CAD build for the part. Positions are in the model's coordinates, mm. Face numbers are marked on the shaded views. A direction names the side the tool comes from. Give positions to 0.01 mm unless a question says otherwise; leave off trailing zeros. Order: outer loops, then holes, each group sorted by start corner. A loop starts at its lowest first (then second) coordinate and runs counter-clockwise, first axis right, second up. Notation, with made-up numbers: M -17,-14.5 L -2,-14.5 A31 ccw -2,17.5 Z; hole C -6,86.5 d4. An arc over 180 degrees is marked long. Put each result on its own line as item: value. Start each with the question number.
1) Drill centre lines: line 1 (Y direction, x = 1, z = 18); line 2 (Y direction, x = 2, z = -5); line 3 (Y direction, x = -14, z = -13.5). Where is each one in solid material? Low to high. Write a range as [from, to].
2) Cut at B-B (y = 19.36). Write the cut outline in (x, z).
3) Cut at C-C (x = -21.5). Write the cut outline in (y, z), and give its area (3 significant figures).
4) Pin check, flat tips, straight feed: pin 1 (4.5 mm diameter, centred on y = 1.5, z = -4, fed in from -X); pin 2 (4 mm diameter, centred on y = 28.685, z = -11.315, fed in from -X); pin 3 (3.5 mm diameter, centred on y = 56.64, z = 18, fed in from +X). Stop position of each tip, or through.
5) Cut at A-A (z = 18). Write the cut outline in (x, y).
6) Cut at D-D (y = 56.64). Write the cut outline in (x, z), and give its area (3 significant figures).
7) Tool access for the marked faces 1, 2 and 3: list every direction of +Z, -Z, +X, -X, +Y, -Y with a clear straight run to the whole face (end or side of a thin tool).
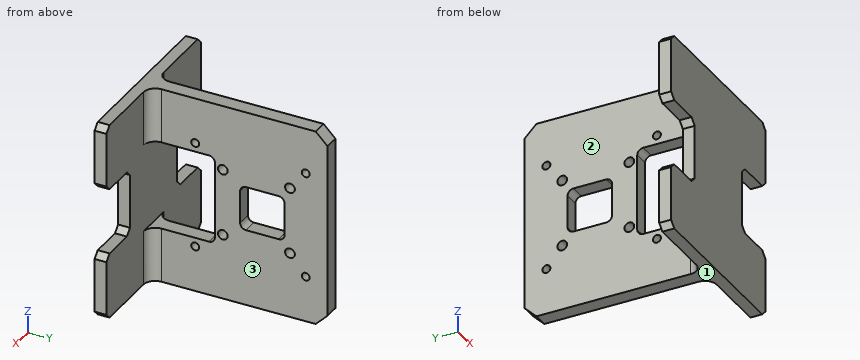
```python
from build123d import *

# Parameters (mm, degrees)
BOSS_EXTRUDE1_DEPTH = 4
SKETCH2_W           = 5
SKETCH2_H           = 67
BOSS_EXTRUDE2_DEPTH = 60
SKETCH3_R           = 1.65
CUT_EXTRUDE1_DEPTH  = 33.5
SKETCH6_R           = 1.35
CUT_EXTRUDE3_DEPTH  = 33.5
SKETCH8_W           = 15
SKETCH8_H           = 15
CUT_EXTRUDE4_DEPTH  = 33.5
SKETCH9_W           = 30
SKETCH9_H           = 22
CUT_EXTRUDE5_DEPTH  = 33.5
FILLET1_R           = 2
FILLET2_R           = 2
CHAMFER1_SIZE       = 2
CHAMFER2_SIZE       = 2
CHAMFER3_SIZE       = 4
FILLET4_R           = 4


with BuildPart() as part:
    # Sketch1 → Boss-Extrude1 (new body)
    with BuildSketch(Plane(origin=(0, 0, 0), x_dir=(1, 0, 0), z_dir=(0, 1, 0))):
        Polygon((-30, 33.5), (30, 33.5), (30, 11.166666667), (15, 11.166666667), (15, -11.166666667), (30, -11.166666667), (30, -33.5), (-30, -33.5), (-30, -11.166666667), (-15, -11.166666667), (-15, 11.166666667), (-30, 11.166666667), align=None)
    extrude(amount=BOSS_EXTRUDE1_DEPTH)

    # Sketch2 → Boss-Extrude2 (add)
    with BuildSketch(Plane(origin=(0, 4, 0), x_dir=(1, 0, 0), z_dir=(0, 1, 0))):
        Rectangle(SKETCH2_W, SKETCH2_H)
    extrude(amount=BOSS_EXTRUDE2_DEPTH)

    # Sketch3 → Cut-Extrude1 (cut, through all)
    with BuildSketch(Plane.ZY.offset(2.5)):
        with Locations((-11.315, 51.315)):
            Circle(SKETCH3_R)
        with Locations((-11.315, 28.685)):
            Circle(SKETCH3_R)
        with Locations((11.315, 28.685)):
            Circle(SKETCH3_R)
        with Locations((11.315, 51.315)):
            Circle(SKETCH3_R)
    extrude(amount=-CUT_EXTRUDE1_DEPTH, mode=Mode.SUBTRACT)

    # Sketch6 → Cut-Extrude3 (cut, through all)
    with BuildSketch(Plane.ZY.offset(2.5)):
        with Locations((-18, 56.64)):
            Circle(SKETCH6_R)
        with Locations((18, 56.64)):
            Circle(SKETCH6_R)
        with Locations((18, 19.36)):
            Circle(SKETCH6_R)
        with Locations((-18, 19.36)):
            Circle(SKETCH6_R)
    extrude(amount=-CUT_EXTRUDE3_DEPTH, mode=Mode.SUBTRACT)

    # Sketch8 → Cut-Extrude4 (cut, through all)
    with BuildSketch(Plane(origin=(2.5, 0, 0), x_dir=(0, 0, -1), z_dir=(1, 0, 0))):
        with Locations((0, 42)):
            Rectangle(SKETCH8_W, SKETCH8_H)
    extrude(amount=-CUT_EXTRUDE4_DEPTH, mode=Mode.SUBTRACT)

    # Sketch9 → Cut-Extrude5 (cut, through all)
    with BuildSketch(Plane(origin=(2.5, 0, 0), x_dir=(0, 0, -1), z_dir=(1, 0, 0))):
        with Locations((0, 15)):
            Rectangle(SKETCH9_W, SKETCH9_H)
    extrude(amount=-CUT_EXTRUDE5_DEPTH, mode=Mode.SUBTRACT)

    # Fillet1
    fillet1_edges = [part.edges().sort_by_distance(p)[0] for p in [
        (0, 26, -15),
        (0, 26, 15),
    ]]
    fillet(fillet1_edges, radius=FILLET1_R)

    # Fillet2
    fillet2_edges = [part.edges().sort_by_distance(p)[0] for p in [
        (0, 49.5, -7.5),
        (0, 34.5, -7.5),
        (0, 34.5, 7.5),
        (0, 49.5, 7.5),
    ]]
    fillet(fillet2_edges, radius=FILLET2_R)

    # Chamfer1
    chamfer1_edges = [part.edges().sort_by_distance(p)[0] for p in [
        (30, 2, -11.166666667),
        (30, 2, 11.166666667),
        (30, 2, 33.5),
        (-30, 2, 33.5),
        (-30, 2, 11.166666667),
        (-30, 2, -11.166666667),
        (-30, 2, -33.5),
        (30, 2, -33.5),
    ]]
    chamfer(chamfer1_edges, length=CHAMFER1_SIZE)

    # Chamfer2
    chamfer2_edges = [part.edges().sort_by_distance(p)[0] for p in [
        (15, 2, -11.166666667),
        (15, 2, 11.166666667),
        (-15, 2, 11.166666667),
        (-15, 2, -11.166666667),
    ]]
    chamfer(chamfer2_edges, length=CHAMFER2_SIZE)

    # Chamfer3
    chamfer3_edges = [part.edges().sort_by_distance(p)[0] for p in [
        (0, 64, -33.5),
        (0, 64, 33.5),
    ]]
    chamfer(chamfer3_edges, length=CHAMFER3_SIZE)

    # Fillet4
    fillet4_edges = [part.edges().sort_by_distance(p)[0] for p in [
        (-2.5, 4, 24.25),
        (2.5, 4, -24.25),
        (2.5, 4, 24.25),
        (-2.5, 4, -24.25),
    ]]
    fillet(fillet4_edges, radius=FILLET4_R)


solid = part.part
```
Solution:
1. line 1: [0, 18.01], [20.71, 55.29], [57.99, 64]
1. line 2: [0, 4], [26, 34.5], [49.5, 64]
1. line 3: [0, 4]
2. outline: M -2.5,-33.5 L 2.5,-33.5 L 2.5,-19.35 L -2.5,-19.35 Z; M -2.5,-16.65 L 2.5,-16.65 L 2.5,-15 L -2.5,-15 Z; M -2.5,15 L 2.5,15 L 2.5,16.65 L -2.5,16.65 Z; M -2.5,19.35 L 2.5,19.35 L 2.5,33.5 L -2.5,33.5 Z
3. outline: M 0,-33.5 L 4,-33.5 L 4,-11.17 L 0,-11.17 Z; M 0,11.17 L 4,11.17 L 4,33.5 L 0,33.5 Z
3. area: 179 mm²
4. pin 1: x = -15
4. pin 2: x = -2.5
4. pin 3: x = 2.5
5. outline: M -30,0 L 30,0 L 30,4 L 6.5,4 A4 cw 2.5,8 L 2.5,18.01 L -2.5,18.01 L -2.5,8 A4 cw -6.5,4 L -30,4 Z; M -2.5,20.71 L 2.5,20.71 L 2.5,55.29 L -2.5,55.29 Z; M -2.5,57.99 L 2.5,57.99 L 2.5,64 L -2.5,64 Z
6. outline: M -2.5,-33.5 L 2.5,-33.5 L 2.5,-19.35 L -2.5,-19.35 Z; M -2.5,-16.65 L 2.5,-16.65 L 2.5,16.65 L -2.5,16.65 Z; M -2.5,19.35 L 2.5,19.35 L 2.5,33.5 L -2.5,33.5 Z
6. area: 308 mm²
7. face 1: -Z, +X, -X, +Y, -Y
7. face 2: +Z, -Z, -X, +Y
7. face 3: +Z, -Z, +X, +Y
